Can you work these out from the model? Positions are in its coordinate system, mm. Round coordinates to 2 decimals unless told otherwise and drop trailing zeros. Order: outer loops, then holes, each group sorted by start corner. A loop starts at its lowest first (then second) coordinate and runs counter-clockwise, first axis right, second up. Notation, with made-up numbers: M -31,40.25 L -9,40.25 A9 cw -9,45.25 Z; hole C -32,42.5 d10. An arc over 180 degrees is marked long. Answer as a JSON object with one key per item and string values. Group by question number.
Autodesk Fusion 360 part; units mm, degrees
sketch "草图1" plane through (0, 0, 0) normal (0, 0, 1) x (1, 0, 0)
  line L0 (-80, -84.3478) -> (-80, 11.2707)
  line L1 (80, -84.3478) -> (80, 8.2588)
  circle A0 centre (-64, -85.6725) radius 1.5
  circle A1 centre (-40, -85.6725) radius 1.5
  circle A2 centre (-64, -55.6725) radius 1.5
  circle A3 centre (-40, -55.6725) radius 1.5
  circle A4 centre (40, -55.6725) radius 1.5
  circle A5 centre (64, -55.6725) radius 1.5
  circle A6 centre (40, -85.6725) radius 1.5
  circle A7 centre (64, -85.6725) radius 1.5
  circle A8 centre (-20.5, 25) radius 1.5
  circle A9 centre (20.5, 25) radius 1.5
  line L2 (-1.5, 45) -> (-1.5, 24)
  arc A10 (-1.5, 24) -> (1.5, 24) centre (0, 24) ccw
  line L3 (1.5, 24) -> (1.5, 45)
  arc A11 (1.5, 45) -> (-1.5, 45) centre (0, 45) ccw
  line L4 (0, 46.5) -> (0, 22.5) construction
  arc A12 (80, 8.2588) -> (-80, 11.2707) centre (-1.119, -49.6781) ccw
  arc A13 (-80, -84.3478) -> (80, -84.3478) centre (0, 112.2701) ccw
  point P0 (0, 50)
  dimension "d4" = 3
  dimension "d7" = 24
  dimension "d8" = 30
  dimension "d9" = 40
  dimension "d10" = 3
  dimension "d11" = 30
  dimension "d14" = 24
  dimension "d15" = -30
  dimension "d16" = 40
  dimension "d17" = 3
  dimension "d22" = 20.5
  dimension "d24" = 20.5
  dimension "d25" = 41
  dimension "d26" = 3
  dimension "d29" = 80
  dimension "d30" = 80
  dimension "d33" = 5
extrude "拉伸1" add sketch "草图1" along normal blind 2
extrude "拉伸2" add sketch "草图1" along normal blind 6
equation "d22 = 19 mm + 1.5 mm"
equation "d25 = 38 mm + 3 mm"
Item 1: Suppose I cut it at D-D, the plane x = 55. Write out the boundary of the cut face in (y, z), and give its area (3 significant figures).
Item 2: I'm going to push flat-ended pins straight in: pin 1 Ø5 at (x, y) = (40, -55.67) entering from +Z; pin 2 Ø2 at (x, z) = (-57, 3.5) entering from -Y. Where does each tip first touch, or does it pass through?
Item 3: Suppose I cut it at A-A, the plane y = 31. Write out the boundary of the cut face in (x, z), and give its area (3 significant figures).
Item 4: Suppose I cut it at B-B, the plane z = 1. State how many separate pieces and enclosed holes the cut face has, and give its area (3 significant figures).
Item 5: I need wall thicknesses on line 1 (Y direction, x = 64, z = 2.15); line 2 (Y direction, x = -64, z = 2.4); line 3 (X direction, y = -54.5, z = 3.6). Which ranges of each line are inside material? Lowest first, please.
Item 6: Suppose I cut it at C-C, the plane x = -25.5. Write out the boundary of the cut face in (y, z), and give its area (3 significant figures).
Item 7: If we mould it in two halves opening along X, with no side actions, what happens to faces 1 (the face through (-1.5, 35, 3)), 2 (the face through (1.148, -99.997, 2.958)), 3 (the face through (-1, -24, 6)), 4 (the face through (1.5, 34, 3))? For each: +X half, -X half, draft (parallel to the pull), parting line (faces both ways), or undercut.
Computed:
{
 "1": {"outline": "M -92.75,0 L 32.71,0 L 32.71,6 L -92.75,6 Z", "area": "753 mm^2"},
 "2": {"pin 1": "stops at z = 6", "pin 2": "stops at y = -92.48"},
 "3": {"outline": "M -59.67,0 L -1.5,0 L -1.5,6 L -59.67,6 Z; M 1.5,0 L 57.43,0 L 57.43,6 L 1.5,6 Z", "area": "685 mm^2"},
 "4": {"separate pieces": "1", "enclosed holes": "11", "area": "21,100 mm^2"},
 "5": {"line 1": "y = -90.12 to -87.17, -84.17 to -57.17, -54.17 to 25.8", "line 2": "y = -90.12 to -87.17, -84.17 to -57.17, -54.17 to 27.67", "line 3": "x = -80 to -64.94, -63.06 to -40.94, -39.06 to 39.06, 40.94 to 63.06, 64.94 to 80"},
 "6": {"outline": "M -98.46,0 L 46.98,0 L 46.98,6 L -98.46,6 Z", "area": "873 mm^2"},
 "7": {"face 1": "undercut", "face 2": "parting line", "face 3": "draft", "face 4": "undercut"}
}
